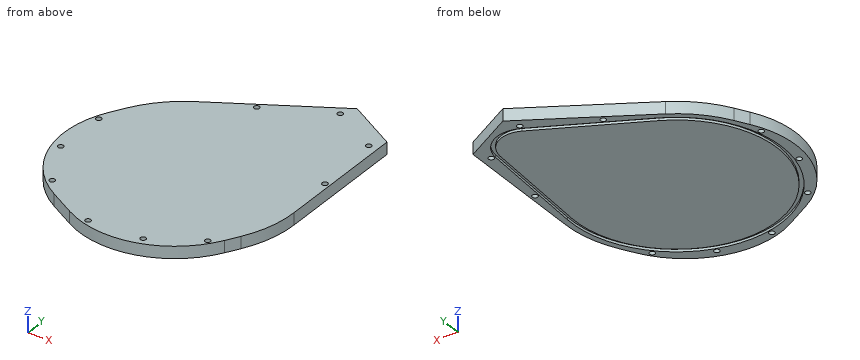
from build123d import *

# Parameters (mm, degrees)
BOSS_EXTRUDE2_DEPTH         = 6.35
F_4_CLEARANCE_HOLE1_D       = 2.9464
CUT_EXTRUDE2_DASH_048_DEPTH = 1.3208
FILLET1_R                   = 50.8


with BuildPart() as part:
    # Sketch3 → Boss-Extrude2 (new body)
    with BuildSketch(Plane(origin=(0.103482409, 1.991370524, 0), x_dir=(1, 0, 0), z_dir=(0, 0, 1))):
        with BuildLine():
            Line((58.7375, 0), (58.7375, 71.178534783))
            Line((58.7375, 71.178534783), (32.273669326, 86.457434546))
            Line((32.273669326, 86.457434546), (-29.36875, 50.868167155))
            ThreePointArc((-29.36875, 50.868167155), (-41.53368456, 41.53368456), (-50.868167155, 29.36875))
            Line((-50.868167155, 29.36875), (-80.236917155, -21.499417155))
            Line((-80.236917155, -21.499417155), (21.499417155, -80.236917155))
            Line((21.499417155, -80.236917155), (50.868167155, -29.36875))
            ThreePointArc((50.868167155, -29.36875), (56.736068222, -15.202383662), (58.7375, 0))
        make_face()
    extrude(amount=BOSS_EXTRUDE2_DEPTH)

    # #4 Clearance Hole1 (through all)
    with Locations(Plane.XY.offset(6.35)):
        with Locations((28.667480209, 80.767509471), (54.04362105, 66.116587726), (-4.272114917, 64.335461198), (-55.5710271, 17.274918559), (-56.146896149, -11.01373469), (-43.178667679, -36.217180003), (-11.345017944, -54.596346246), (16.965920195, -53.225438887), (41.176678022, -38.582395037), (56.282847372, 29.37403742)):
            Hole(F_4_CLEARANCE_HOLE1_D / 2)

    # Sketch6 → Cut-Extrude2 - dash 048 (cut)
    with BuildSketch(Plane(origin=(0.103482409, 1.991370524, 0), x_dir=(1, 0, 0), z_dir=(0, 0, 1))):
        with BuildLine():
            Line((55.672086916, 3.229866087), (52.009478425, 63.620294443))
            ThreePointArc((52.009478425, 63.620294443), (44.021350779, 76.247216167), (29.092051971, 76.851676775))
            Line((29.092051971, 76.851676775), (-25.038897376, 49.828374594))
            ThreePointArc((-25.038897376, 49.828374594), (-27.88285, -48.29451286), (55.672086916, 3.229866087))
        make_face()
        with BuildLine():
            Line((53.466162602, 3.099012969), (49.805143409, 63.46323641))
            ThreePointArc((49.805143409, 63.46323641), (42.916450779, 74.33347323), (30.058203233, 74.864137637))
            Line((30.058203233, 74.864137637), (-24.049257344, 47.852561541))
            ThreePointArc((-24.049257344, 47.852561541), (-26.77795, -46.380769923), (53.466162602, 3.099012969))
        make_face(mode=Mode.SUBTRACT)
    extrude(amount=CUT_EXTRUDE2_DASH_048_DEPTH, mode=Mode.SUBTRACT)

    # Fillet1
    fillet1_edges = [part.edges().sort_by_distance(p)[0] for p in [
        (21.602899564, -78.245546631, 3.175),
        (-80.133434745, -19.508046631, 3.175),
    ]]
    fillet(fillet1_edges, radius=FILLET1_R)


solid = part.part
Input: part model. Units: mm. Frame: model coordinates. Round coordinates to 2 decimals unless told otherwise and drop trailing zeros. Write each loop counter-clockwise with the first axis right and the second up, starting at its lowest first coordinate (ties: lowest second). Pieces come first, ordered by that corner, then holes.
1) Cut plane A-A (z = 4.75). Count the separate pieces of the cut face and the enclosed holes in it, then the cut area to 3 significant figures.
2) Ray query, L1, parallel to Y at x = -36, z = 1.25; L2, parallel to Y at x = -29.5, z = 1; L3, parallel to Y at x = 42.5, z = 1.25. Return the intervals inside material, ascending.
3) Cut plane C-C (x = 12). Return the cut outline in (y, z).
4) Cut plane B-B (y = 36). Return the cut outline in (x, z).
5) Contact query for flat-ended pins moving along their axis: P1, Ø1.5, axis at x = 45.5, z = 1, coming from the -Y side; P2, Ø1.5, axis at x = 16.5, z = 2.5, coming from the +Y side; P3, Ø4, axis at x = -11.35, y = -54.6, coming from the -Z side. Output: stop coordinate, or through.
Geometry says:
1. separate pieces: 1
1. enclosed holes: 10
1. area: 13,100 mm2
2. L1: y = -44.99 to -40.51, -37.57 to 41.55, 44.49 to 48.32
2. L2: y = -48.74 to -45.27, -42.64 to 46.62, 49.25 to 52.72
2. L3: y = -40.81 to -39.23, -37.93 to -34.23, -30.73 to 76.61, 79.06 to 82.6
3. outline: (-58.85, 0) - (-52.49, 0) - (-52.49, 1.32) - (-50.23, 1.32) - (-50.23, 0) - (67.79, 0) - (67.79, 1.32) - (70.26, 1.32) - (70.26, 0) - (76.68, 0) - (76.68, 6.35) - (-58.85, 6.35) - close
4. outline: (-47.79, 0) - (-44.09, 0) - (-44.09, 1.32) - (-41.27, 1.32) - (-41.27, 0) - (51.7, 0) - (51.7, 1.32) - (53.91, 1.32) - (53.91, 0) - (58.84, 0) - (58.84, 6.35) - (-47.79, 6.35) - close
5. P1: stops at y = -37.81
5. P2: stops at y = 79.72
5. P3: stops at z = 0
